The drawing under review shows one solid part. Ordinate dimensions are in mm from its lowest x, y, z. A direction names the side the tool comes from. Give positions to 0.01 mm unless a question says otherwise; leave off trailing zeros. Write each loop counter-clockwise with the first axis right and the second up, starting at its lowest first coordinate (ties: lowest second). Pieces come first, ordered by that corner, then holes. Notation, with made-up numbers: (38, 65.25) -> (54, 65.25) arc R31 ccw to (54, 89.25) -> close; hole circle Ø3 at (-29.5, 79). An arc over 180 degrees is marked (long way). Write item = value, one per line.
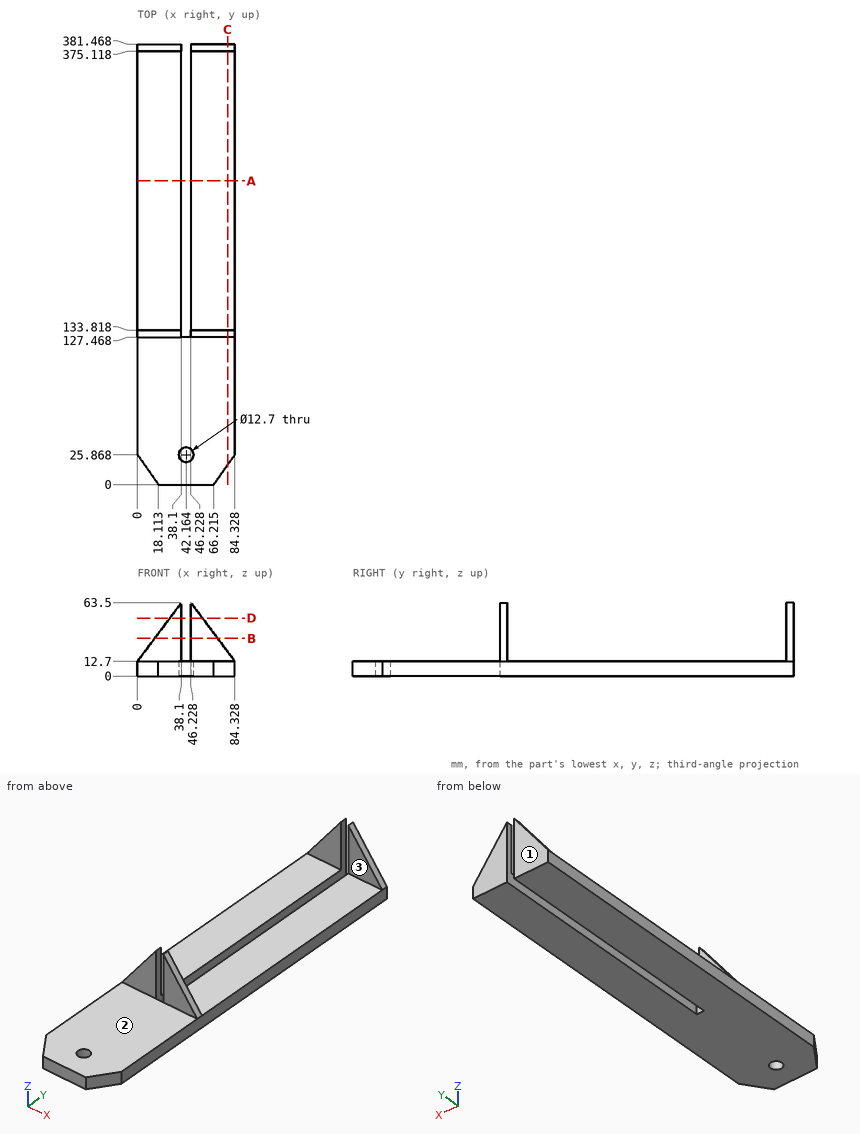
(1) Take a section at C-C (x = 78). Write out the cut boundary in (y, z), plus the area to 3 significant figures.
Answers below:
outline = (16.83, 0) -> (381.47, 0) -> (381.47, 21.14) -> (375.12, 21.14) -> (375.12, 12.7) -> (133.82, 12.7) -> (133.82, 21.14) -> (127.47, 21.14) -> (127.47, 12.7) -> (16.83, 12.7) -> close
area = 4,740 mm^2
(2) Take a section at A-A (y = 263). Write out the cut boundary in (x, z), plus the area to 3 significant figures.
Answers below:
outline = (0, 0) -> (38.1, 0) -> (38.1, 12.7) -> (0, 12.7) -> close; (46.23, 0) -> (84.33, 0) -> (84.33, 12.7) -> (46.23, 12.7) -> close
area = 968 mm^2
(3) Tool access review of the marked faces 1, 2 and 3: name each direction out of +Z, -Z, +X, -X, +Y, -Y from which nothing blocks a thin tool from reaching the whole face with its end or side.
Answers below:
face_1 = +Z, -Z, +X, -X, +Y
face_2 = +Z, +X, -X, -Y
face_3 = +Z, +X, -X
(4) To check wall thickness, follow probe 1 along X at (y, z) = (332.5, 12); probe 2 along Y at (x, z) = (63, 20); probe 3 along Z at (x, y) = (19, 224). State the ranges of each line that lie inside material, in increasing order.
Answers below:
probe_1 = 0 to 38.1, 46.23 to 84.33
probe_2 = 127.47 to 133.82, 375.12 to 381.47
probe_3 = 0 to 12.7
(5) For pin 1 (5 mm diameter, centred on x = 69.5, z = 34.5, fed in from -Y); pin 2 (2 mm diameter, centred on x = 49, y = 81.5, fed in from -Z); pin 3 (11.5 mm diameter, centred on x = 25.5, y = 251, fed in from +Z), all flat-tipped, find the tip position at first contact; note any pin that passes through.
Answers below:
pin_1 = 127.47
pin_2 = 0
pin_3 = 12.7
(6) Take a section at D-D (z = 50). Write out the cut boundary in (x, y) (1 decimal).
Answers below:
outline = (28, 127.5) -> (38.1, 127.5) -> (38.1, 133.8) -> (28, 133.8) -> close; (28, 375.1) -> (38.1, 375.1) -> (38.1, 381.5) -> (28, 381.5) -> close; (46.2, 127.5) -> (56.4, 127.5) -> (56.4, 133.8) -> (46.2, 133.8) -> close; (46.2, 375.1) -> (56.4, 375.1) -> (56.4, 381.5) -> (46.2, 381.5) -> close
(7) Take a section at B-B (z = 32.5). Write out the cut boundary in (x, y).
Answers below:
outline = (14.85, 127.47) -> (38.1, 127.47) -> (38.1, 133.82) -> (14.85, 133.82) -> close; (14.85, 375.12) -> (38.1, 375.12) -> (38.1, 381.47) -> (14.85, 381.47) -> close; (46.23, 127.47) -> (69.48, 127.47) -> (69.48, 133.82) -> (46.23, 133.82) -> close; (46.23, 375.12) -> (69.48, 375.12) -> (69.48, 381.47) -> (46.23, 381.47) -> close
